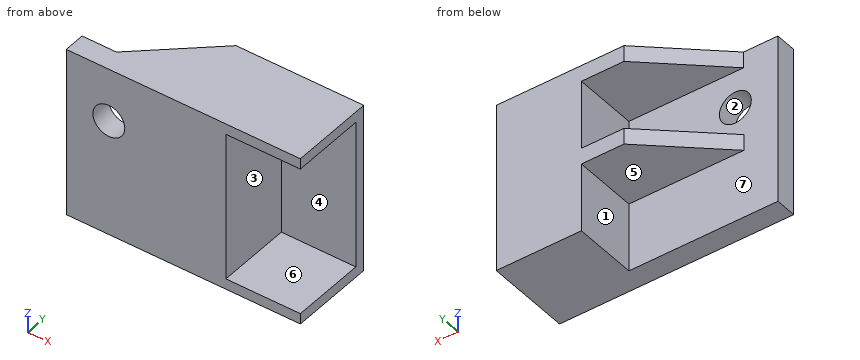
from build123d import *

# Parameters (mm, degrees)
SKETCH1_W            = 139.7
SKETCH1_H            = 101.6
BOSS_EXTRUDE1_DEPTH  = 12.7
SKETCH2_W            = 44.45
SKETCH2_H            = 6.35
BOSS_EXTRUDE2_DEPTH  = 31.75
SKETCH3_W            = 44.45
SKETCH3_H            = 6.35
BOSS_EXTRUDE3_DEPTH  = 31.75
SKETCH4_W            = 6.35
SKETCH4_H            = 101.6
BOSS_EXTRUDE4_DEPTH  = 31.75
SKETCH5_W            = 50.8
SKETCH5_H            = 101.6
BOSS_EXTRUDE5_DEPTH  = 6.35
SKETCH7_W            = 44.45
SKETCH7_H            = 88.9
BOSS_EXTRUDE7_DEPTH  = 12.7
SKETCH9_W            = 44.45
SKETCH9_H            = 88.9
CUT_EXTRUDE1_DEPTH   = 12.7
SKETCH10_W           = 25.218134922
SKETCH10_H           = 9.68567434
BOSS_EXTRUDE8_DEPTH  = 38.1
SKETCH11_W           = 25.4
SKETCH11_H           = 9.652
BOSS_EXTRUDE9_DEPTH  = 38.1
SKETCH12_R           = 9.525
CUT_EXTRUDE2_DEPTH   = 38.1
SKETCH13_W           = 43.179728204
SKETCH13_H           = 9.652
BOSS_EXTRUDE10_DEPTH = 38.1
SKETCH14_W           = 43.18
SKETCH14_H           = 9.68567434
BOSS_EXTRUDE11_DEPTH = 38.1
CUT_EXTRUDE8_START   = -9.68567434
CUT_EXTRUDE8_DEPTH   = 9.68567434
CUT_EXTRUDE10_DEPTH  = 38.1


# Read off the part's stored shape, not the designer's step: Cut-Extrude8
with BuildPart() as part:
    # Sketch1 → Boss-Extrude1 (new body)
    with BuildSketch(Plane(origin=(0, 0, 0), x_dir=(1, 0, 0), z_dir=(0, 1, 0))):
        with Locations((69.85, 50.8)):
            Rectangle(SKETCH1_W, SKETCH1_H)
    extrude(amount=BOSS_EXTRUDE1_DEPTH)

    # Sketch2 → Boss-Extrude2 (add)
    with BuildSketch(Plane(origin=(0, 12.7, 0), x_dir=(1, 0, 0), z_dir=(0, 1, 0))):
        with Locations((117.475, 3.175)):
            Rectangle(SKETCH2_W, SKETCH2_H)
    extrude(amount=BOSS_EXTRUDE2_DEPTH)

    # Sketch3 → Boss-Extrude3 (add)
    with BuildSketch(Plane(origin=(0, 12.7, 0), x_dir=(1, 0, 0), z_dir=(0, 1, 0))):
        with Locations((117.475, 98.425)):
            Rectangle(SKETCH3_W, SKETCH3_H)
    extrude(amount=BOSS_EXTRUDE3_DEPTH)

    # Sketch4 → Boss-Extrude4 (add)
    with BuildSketch(Plane(origin=(0, 12.7, 0), x_dir=(1, 0, 0), z_dir=(0, 1, 0))):
        with Locations((92.075, 50.8)):
            Rectangle(SKETCH4_W, SKETCH4_H)
    extrude(amount=BOSS_EXTRUDE4_DEPTH)

    # Sketch5 → Boss-Extrude5 (add)
    with BuildSketch(Plane(origin=(0, 44.45, 0), x_dir=(1, 0, 0), z_dir=(0, 1, 0))):
        with Locations((114.3, 50.8)):
            Rectangle(SKETCH5_W, SKETCH5_H)
    extrude(amount=BOSS_EXTRUDE5_DEPTH)

    # Sketch7 → Boss-Extrude7 (add)
    with BuildSketch(Plane(origin=(0, 12.7, 0), x_dir=(1, 0, 0), z_dir=(0, 1, 0))):
        with Locations((117.475, 50.8)):
            Rectangle(SKETCH7_W, SKETCH7_H)
    extrude(amount=-BOSS_EXTRUDE7_DEPTH)

    # Sketch9 → Cut-Extrude1 (cut)
    with BuildSketch(Plane(origin=(0, 12.7, 0), x_dir=(1, 0, 0), z_dir=(0, 1, 0))):
        with Locations((117.475, 50.8)):
            Rectangle(SKETCH9_W, SKETCH9_H)
    extrude(amount=-CUT_EXTRUDE1_DEPTH, mode=Mode.SUBTRACT)

    # Sketch10 → Boss-Extrude8 (add)
    with BuildSketch(Plane(origin=(0, 12.7, 0), x_dir=(1, 0, 0), z_dir=(0, 1, 0))):
        with Locations((76.290932539, 4.84283717)):
            Rectangle(SKETCH10_W, SKETCH10_H)
    extrude(amount=BOSS_EXTRUDE8_DEPTH)

    # Sketch11 → Boss-Extrude9 (add)
    with BuildSketch(Plane(origin=(0, 12.7, 0), x_dir=(1, 0, 0), z_dir=(0, 1, 0))):
        with Locations((76.2, 55.693142425)):
            Rectangle(SKETCH11_W, SKETCH11_H)
    extrude(amount=BOSS_EXTRUDE9_DEPTH)

    # Sketch12 → Cut-Extrude2 (cut)
    with BuildSketch(Plane(origin=(0, 12.7, 0), x_dir=(1, 0, 0), z_dir=(0, 1, 0))):
        with Locations(Location((25.4, 31.75, 0), (0, 0, 270))):
            Circle(SKETCH12_R)
    extrude(amount=-CUT_EXTRUDE2_DEPTH, mode=Mode.SUBTRACT)

    # Sketch13 → Boss-Extrude10 (add)
    with BuildSketch(Plane(origin=(0, 12.7, 0), x_dir=(1, 0, 0), z_dir=(0, 1, 0))):
        with Locations((41.910135898, 55.693142425)):
            Rectangle(SKETCH13_W, SKETCH13_H)
    extrude(amount=BOSS_EXTRUDE10_DEPTH)

    # Sketch14 → Boss-Extrude11 (add)
    with BuildSketch(Plane(origin=(0, 12.7, 0), x_dir=(1, 0, 0), z_dir=(0, 1, 0))):
        with Locations((42.091865078, 4.84283717)):
            Rectangle(SKETCH14_W, SKETCH14_H)
    extrude(amount=BOSS_EXTRUDE11_DEPTH)

    # Cut-Extrude8 outline → Cut-Extrude8 (cut)
    with BuildSketch(Plane.XY.offset(CUT_EXTRUDE8_START)):
        Polygon((20.501865078, 50.8), (20.501865078, 12.7), (63.500271796, 50.8), align=None)
    extrude(amount=CUT_EXTRUDE8_DEPTH, mode=Mode.SUBTRACT)

    # Sketch16 → Cut-Extrude10 (cut)
    with BuildSketch(Plane.XY.offset(-50.867142425)):
        Polygon((20.320271796, 12.7), (20.320271796, 50.8), (63.500271796, 50.8), align=None)
    extrude(amount=-CUT_EXTRUDE10_DEPTH, mode=Mode.SUBTRACT)


solid = part.part
The listing builds one solid part. Answer for the finished solid, in the listing's coordinates (mm). Face numbers are marked on the shaded views. A direction names the side the tool comes from. Coordinates: 2 decimals unless noted, no trailing zeros. Write each loop counter-clockwise with the first axis right and the second up, starting at its lowest first coordinate (ties: lowest second). Pieces come first, ordered by that corner, then holes. Notation, with made-up numbers: M 24.5,-27 L 63.5,-27 A28 cw 63.5,9 Z; hole C 59.25,4 d8. An arc over 180 degrees is marked long. Put each result on its own line as item: value. Start each with the question number.
1. Which of the six approach directions +Z, -Z, +X, -X, +Y, -Y give full straight-line access (tool end or side, diameter ignored) to the marked faces 5, 6 and 7?
2. A cutting plane is placed at D-D on z = -82. Write down the section's boundary in (x, y), then the cut area to 3 significant figures.
3. For a pull along X with two mould halves and no side action, classify the marked faces 1, 2, 3 and 4 as pulls with the +X half, pulls with the -X half, needs draft (parallel to the pull), parting line crosses it, or undercut.
4. A cutting plane is placed at B-B on y = 11. Write down the section's boundary in (x, z) (3 decimals).
5. A cutting plane is placed at C-C on x = 25.4. Write down the section's boundary in (y, z) (3 decimals).
6. A cutting plane is placed at A-A on z = -31.75. Write down the section's boundary in (x, y) (3 decimals), then the cut area to 3 significant figures.
7. Consider line 1 (Z direction, x = 124.5, y = 15); line 2 (Z direction, x = 25, y = 5); line 3 (X direction, y = 8.5, z = -31.75) (3 decimals). Determine where each line is inside the solid, lowest interval first. Write a range as from..to.
8. Flat-ended cylindrical pins translate along their axes: P1, Ø5, axis at y = 9, z = -55.5, coming from the +X side; P2, Ø8, axis at y = 32, z = -67.5, coming from the -X side; P3, Ø1.5, axis at x = 14, z = -21, coming from the +Y side. Find the tip coordinate at first contact, or state that the pin passes through.
Resolved:
1. face 5: -Z, -X, +Y
1. face 6: +X, -Y
1. face 7: -X, +Y
2. outline: M 0,0 L 95.25,0 L 95.25,44.45 L 139.7,44.45 L 139.7,50.8 L 88.9,50.8 L 88.9,12.7 L 0,12.7 Z
2. area: 1,730 mm2
3. face 1: pulls with the -X half
3. face 2: undercut
3. face 3: pulls with the +X half
3. face 4: needs draft
4. outline: M 0,-101.6 L 139.7,-101.6 L 139.7,-95.25 L 95.25,-95.25 L 95.25,-6.35 L 139.7,-6.35 L 139.7,0 L 0,0 Z; hole C 25.4,-31.75 d19.05
5. outline: M 0,-101.6 L 12.7,-101.6 L 12.7,-60.519 L 17.182,-60.519 L 17.182,-50.867 L 12.7,-50.867 L 12.7,-41.275 L 0,-41.275 Z; M 0,-22.225 L 12.7,-22.225 L 12.7,-9.686 L 17.04,-9.686 L 17.04,0 L 0,0 Z
6. outline: M 0,0 L 15.875,0 L 15.875,12.7 L 0,12.7 Z; M 34.925,0 L 95.25,0 L 95.25,44.45 L 139.7,44.45 L 139.7,50.8 L 88.9,50.8 L 88.9,12.7 L 34.925,12.7 Z
6. area: 1,490 mm2
7. line 1: z = -101.6..-95.25, -6.35..0
7. line 2: z = -101.6..-41.27, -22.23..0
7. line 3: x = 0..15.875, 34.925..95.25
8. P1: stops at x = 95.25
8. P2: stops at x = 88.9
8. P3: stops at y = 12.7
